Geometry: final body of the model. Coordinates: model frame, mm. Face numbers are marked on the shaded views. A direction names the side the tool comes from. Give positions to 0.01 mm unless a question says otherwise; leave off trailing zeros. Loops run counter-clockwise (first coordinate to the right, second up) from the corner with the lowest first, then second, coordinate; pieces in that order, holes last. Notation, with made-up numbers: (1, 5) -> (32, 5) arc R14 ccw to (32, 23) -> close; hole circle Ø5 at (19.5, 40.5). An arc over 180 degrees is marked (long way). One line per item, written item: value. Start each with the question number.
Autodesk Inventor part; units mm, degrees
ref_plane "YZ Plane" through (0, 0, 0) normal (1, 0, 0) x (0, 1, 0)
ref_plane "XZ Plane" through (0, 0, 0) normal (0, 1, 0) x (-1, 0, 0)
ref_plane "XY Plane" through (0, 0, 0) normal (0, 0, 1) x (1, 0, 0)
sketch "スケッチ1" plane through (0, 0, 0) normal (0, 1, 0) x (-1, 0, 0)
  line L0 (0, 0) -> (-90, 0)
  line L1 (-90, 0) -> (-90, 50)
  line L2 (0, 50) -> (0, 0)
  line L3 (0, 0) -> (-5, 0)
  line L4 (-5, 0) -> (-5, 50)
  line L5 (-5, 0) -> (-90, 0)
  line L6 (-90, 0) -> (-85, 0)
  line L7 (-85, 0) -> (-85, 50)
  arc A0 (-85, 50) -> (-5, 50) centre (-45, 50) ccw
  line L8 (0, 0) -> (0, 10)
  line L9 (0, 10) -> (-90, 10)
  circle A1 centre (-45, 50) radius 45
  line L10 (-90, 5) -> (0, 5)
  line L11 (-90, 50) -> (-85, 50)
  line L12 (-5, 50) -> (0, 50)
  line L13 (0, 0) -> (-90, 0)
  line L14 (-90, 0) -> (-90, 5)
  line L15 (-90, 5) -> (0, 5)
  line L16 (0, 5) -> (0, 0)
  dimension "d0" = 90
  dimension "d1" = 50
  dimension "d2" = 5
  dimension "d3" = 85
  dimension "d4" = 5
  dimension "d5" = 80
  dimension "d6" = 10
  dimension "d7" = 90
extrude "押し出し1" add sketch "スケッチ1" along normal blind 230 contours L0 L4 L10 L2 | L0 L7 L10 L4 | L10 L4 L9 L2 | L0 L1 L10 L7 | L10 A1 L9 L4 | L9 L4 A1 L2 | L10 L1 L9 L7 | L7 L9 A1 L10 | L9 A1 L4 | A1 L9 | A1 L4 L12 | L9 L1 A1 L7 | L7 A1 L9 | A1 L9 A0 L4 | A1 L7 A0 L9 | L11 L7 A1
sketch "スケッチ2" plane through (0, 0, 0) normal (0, -1, 0) x (1, 0, 0)
  line L0 (0, 0) -> (0, 50)
  line L1 (90, 0) -> (0, 0)
  line L2 (90, 50) -> (90, 0)
  line L3 (85, 50) -> (90, 50)
  arc A0 (5, 50) -> (85, 50) centre (45, 50) ccw
  line L4 (0, 50) -> (5, 50)
  arc A1 (5, 23.467) -> (85, 23.467) centre (45, 50) ccw
  line L5 (0, 5) -> (90, 5)
  line L6 (5, 23.467) -> (5, 5)
  line L7 (85, 23.467) -> (85, 5)
  dimension "d29" = 48
extrude "押し出し2" cut sketch "スケッチ2" against normal blind 225 contours L6 A1 L5 | L5 A1 L7
sketch "スケッチ3" plane through (0, 230, 0) normal (0, 1, 0) x (1, 0, 0)
  arc A0 (85, -50) -> (5, -50) centre (45, -50) ccw
  line L0 (90, -50) -> (90, 0)
  line L1 (0, -50) -> (5, -50)
  arc A1 (85, -50) -> (5, -50) centre (45, -50) ccw
  line L2 (5, -50) -> (85, -50)
extrude "押し出し3" add sketch "スケッチ3" against normal blind 5
sketch "スケッチ4" plane through (90, 0, 50) normal (1, 0, 0) x (0, 0, -1)
  line L0 (0, 0) -> (50, 0)
  line L1 (0, 0) -> (0, 230)
  line L2 (25, 0) -> (25, 65)
  line L3 (25, 65) -> (25, 75)
  line L4 (25, 75) -> (25, 215)
  line L5 (25, 215) -> (25, 225)
  line L6 (0, 65) -> (40, 65)
  line L7 (40, 65) -> (40, 75)
  line L8 (40, 75) -> (0, 75)
  line L9 (0, 75) -> (0, 65)
  line L10 (0, 215) -> (40, 215)
  line L11 (40, 215) -> (40, 225)
  line L12 (40, 225) -> (0, 225)
  line L13 (0, 225) -> (0, 215)
  dimension "d16" = 65
  dimension "d17" = 10
  dimension "d18" = 140
  dimension "d19" = 10
  dimension "d20" = 40
extrude "押し出し4" cut sketch "スケッチ4" against normal blind 90 contours L1 L8 L3 L6 | L3 L8 L7 L6 | L1 L12 L5 L10 | L5 L12 L11 L10
sketch "スケッチ6" plane through (90, 0, 50) normal (1, 0, 0) x (0, 0, -1)
  line L0 (0, 230) -> (50, 230)
  line L1 (50, 230) -> (37.5, 251.6506)
  line L2 (50, 230) -> (110, 230) construction
  line L3 (0, 230) -> (37.5, 251.6506)
  line L4 (0, 230) -> (43.3013, 230) construction
  dimension "d32" = 120
  dimension "d33" = 30
extrude "押し出し6" add sketch "スケッチ6" against normal blind 90
sketch "スケッチ9" plane through (0, 0, 0) normal (-1, 0, 0) x (0, 0, 1)
  line L0 (10, 225) -> (50, 225)
  line L1 (50, 225) -> (50, 230)
  line L2 (50, 230) -> (12.5, 251.6506)
  line L3 (12.5, 251.6506) -> (0, 230)
  line L4 (0, 0) -> (0, 230)
  line L5 (0, 0) -> (50, 0)
  line L6 (50, 0) -> (50, 65)
  line L7 (50, 65) -> (10, 65)
  line L8 (10, 65) -> (10, 75)
  line L9 (10, 75) -> (50, 75)
  line L10 (50, 75) -> (50, 215)
  line L11 (50, 215) -> (10, 215)
  line L12 (10, 215) -> (10, 225)
  line L13 (12.5, 251.6506) -> (0, 230)
  line L14 (0, 230) -> (-132.7906, 0)
  line L15 (0, 145) -> (-49.0748, 145)
  line L16 (0, 115) -> (-66.3953, 115)
  dimension "d45" = 30
sketch "スケッチ10" plane through (0, 0, 0) normal (-1, 0, 0) x (0, 0, 1)
  line L0 (10, 225) -> (50, 225)
  line L1 (50, 225) -> (50, 230)
  line L2 (50, 230) -> (12.5, 251.6506)
  line L3 (12.5, 251.6506) -> (0, 230)
  line L4 (0, 0) -> (0, 230)
  line L5 (0, 0) -> (50, 0)
  line L6 (50, 0) -> (50, 65)
  line L7 (50, 65) -> (10, 65)
  line L8 (10, 65) -> (10, 75)
  line L9 (10, 75) -> (50, 75)
  line L10 (50, 75) -> (50, 215)
  line L11 (50, 215) -> (10, 215)
  line L12 (10, 215) -> (10, 225)
  line L13 (12.5, 251.6506) -> (-87.5, 78.4456)
  line L14 (-87.5, 78.4456) -> (50, 0)
sketch "スケッチ12" plane through (90, 0, 50) normal (1, 0, 0) x (0, 0, -1)
  line L0 (50, 0) -> (50, 230)
  line L1 (40, 225) -> (40, 215)
  line L2 (0, 215) -> (0, 75)
  line L3 (0, 145) -> (50, 145)
  line L4 (32.5, 175) -> (17.5, 175)
  line L5 (17.5, 175) -> (17.5, 115)
  line L6 (17.5, 115) -> (32.5, 115)
  line L7 (32.5, 115) -> (32.5, 175)
  line L8 (32.5, 175) -> (17.5, 115) construction
  line L9 (17.5, 175) -> (32.5, 115) construction
  line L10 (17.5, 145) -> (32.5, 145)
  line L11 (32.5, 145) -> (32.5, 115)
  line L12 (32.5, 115) -> (17.5, 115)
  line L13 (17.5, 115) -> (17.5, 145)
  point P0 (25, 145)
  dimension "d59" = 15
  dimension "d60" = 60
extrude "押し出し8" cut sketch "スケッチ12" against normal blind 2.5 contours L3 L7 L6 L5
sketch "スケッチ13" plane through (0, 0, 0) normal (-1, 0, 0) x (0, 0, 1)
  line L0 (0, 0) -> (0, 230)
  line L1 (50, 75) -> (50, 215)
  line L2 (50, 145) -> (0, 145)
  line L3 (17.5, 175) -> (32.5, 175)
  line L4 (32.5, 175) -> (32.5, 115)
  line L5 (32.5, 115) -> (17.5, 115)
  line L6 (17.5, 115) -> (17.5, 175)
  line L7 (17.5, 175) -> (32.5, 115) construction
  line L8 (32.5, 175) -> (17.5, 115) construction
  line L9 (17.5, 145) -> (32.5, 145)
  line L10 (32.5, 145) -> (32.5, 115)
  line L11 (32.5, 115) -> (17.5, 115)
  line L12 (17.5, 115) -> (17.5, 145)
  point P0 (25, 145)
  dimension "d63" = 15
  dimension "d64" = 60
extrude "押し出し9" cut sketch "スケッチ13" against normal blind 2.5 contours L4 L5 L6 L2
sketch "スケッチ14" plane through (90, 0, 0) normal (0, 0, -1) x (-1, 0, 0)
  line L0 (90, 0) -> (90, 230)
  line L1 (0, 0) -> (0, 230)
  line L2 (0, 145) -> (90, 145)
  line L3 (37.5, 170) -> (52.5, 170)
  line L4 (52.5, 170) -> (52.5, 120)
  line L5 (52.5, 120) -> (37.5, 120)
  line L6 (37.5, 120) -> (37.5, 170)
  line L7 (37.5, 170) -> (52.5, 120) construction
  line L8 (52.5, 170) -> (37.5, 120) construction
  line L9 (37.5, 145) -> (52.5, 145)
  line L10 (52.5, 145) -> (52.5, 170)
  line L11 (52.5, 170) -> (37.5, 170)
  line L12 (37.5, 170) -> (37.5, 145)
  point P0 (45, 145)
  dimension "d67" = 15
  dimension "d70" = 25
extrude "押し出し10" cut sketch "スケッチ14" against normal blind 5 contours L6 L3 L4 L2
sketch "スケッチ16" plane through (90, 0, 0) normal (0, 0, -1) x (-1, 0, 0)
  line L0 (52.5, 170) -> (52.5, 145)
  line L1 (52.5, 145) -> (37.5, 145)
  line L2 (37.5, 145) -> (37.5, 170)
  line L3 (90, 0) -> (90, 230)
  line L4 (0, 0) -> (0, 230)
  line L5 (0, 145) -> (90, 145)
  line L6 (0, 160) -> (37.5, 157.5)
  line L7 (52.5, 157.5) -> (90, 157.5)
  line L8 (18.75, 158.75) -> (18.75, 145)
  line L9 (71.25, 145) -> (71.25, 157.5)
  line L10 (11.25, 175) -> (26.25, 175)
  line L11 (26.25, 175) -> (26.25, 115)
  line L12 (26.25, 115) -> (11.25, 115)
  line L13 (11.25, 115) -> (11.25, 175)
  line L14 (11.25, 175) -> (26.25, 115) construction
  line L15 (26.25, 175) -> (11.25, 115) construction
  line L16 (11.25, 115) -> (26.25, 115)
  line L17 (26.25, 115) -> (26.25, 175)
  line L18 (26.25, 175) -> (11.25, 175)
  line L19 (11.25, 175) -> (11.25, 115)
  line L20 (45, 145) -> (45, 125)
  line L21 (78.75, 175) -> (63.75, 175)
  line L22 (63.75, 115) -> (78.75, 115)
  line L23 (78.75, 175) -> (78.75, 115)
  line L24 (63.75, 115) -> (63.75, 175)
  line L25 (63.75, 175) -> (78.75, 175)
  line L26 (78.75, 175) -> (78.75, 115)
  line L27 (78.75, 115) -> (63.75, 115)
  line L28 (63.75, 115) -> (63.75, 175)
  line L29 (11.25, 115) -> (26.25, 115)
  line L30 (26.25, 115) -> (26.25, 175)
  line L31 (26.25, 175) -> (11.25, 175)
  line L32 (11.25, 175) -> (11.25, 115)
  dimension "d71" = 15
  dimension "d72" = 60
  dimension "d73" = 20
extrude "押し出し11" cut sketch "スケッチ16" against normal blind 3 contours L24 L21 L23 L7 | L7 L9 L5 L24 | L5 L23 L22 L24 | L7 L23 L5 L9 | L11 L12 L13 L5 | L5 L8 L6 L11 | L6 L13 L10 L11 | L5 L13 L6 L8
sketch "スケッチ17" plane through (37.5, 145, 0) normal (0, 1, 0) x (1, 0, 0)
  line L0 (-57.7643, 16.522) -> (69.053, 16.522)
  line L1 (69.053, 16.522) -> (69.053, -65.9751)
  line L2 (69.053, -65.9751) -> (-57.7643, -65.9751)
  line L3 (-57.7643, -65.9751) -> (-57.7643, 16.522)
  point P0 (-37.5, 0)
extrude "押し出し12" cut sketch "スケッチ17" against normal blind 180
sketch "スケッチ18" plane through (0, 215, 10) normal (-1, 0, 0) x (0, 0, 1)
  line L0 (-10, -70) -> (40, -70)
  line L1 (7.5, -40) -> (22.5, -40)
  line L2 (22.5, -40) -> (22.5, -100)
  line L3 (22.5, -100) -> (7.5, -100)
  line L4 (7.5, -100) -> (7.5, -40)
  line L5 (7.5, -40) -> (22.5, -100) construction
  line L6 (22.5, -40) -> (7.5, -100) construction
  point P0 (-10, -215)
  point P1 (15, -70)
  dimension "d78" = 15
  dimension "d79" = 60
extrude "押し出し13" add sketch "スケッチ18" against normal blind 2.5
sketch "スケッチ19" plane through (90, 215, 10) normal (1, 0, 0) x (0, 0, -1)
  line L0 (-40, -70) -> (10, -70)
  line L1 (-22.5, -40) -> (-7.5, -40)
  line L2 (-7.5, -40) -> (-7.5, -100)
  line L3 (-7.5, -100) -> (-22.5, -100)
  line L4 (-22.5, -100) -> (-22.5, -40)
  line L5 (-22.5, -40) -> (-7.5, -100) construction
  line L6 (-7.5, -40) -> (-22.5, -100) construction
  point P0 (10, -215)
  point P1 (-15, -70)
  dimension "d82" = 15
  dimension "d83" = 60
extrude "押し出し14" add sketch "スケッチ19" against normal blind 2.5
sketch "スケッチ20" plane through (90, 230, 0) normal (0, 0.5, -0.866) x (-1, 0, 0)
  line L0 (0, 0) -> (0, 25)
  line L1 (0, 0) -> (90, 0)
  line L2 (90, 25) -> (90, 0)
  line L3 (0, 25) -> (90, 25)
  line L4 (0, 12.5) -> (90, 12.5)
  line L5 (45, 12.5) -> (45, 25)
  line L6 (45, 12.5) -> (45, 0)
  line L7 (22.5, 18.5) -> (67.5, 18.5)
  line L8 (67.5, 18.5) -> (67.5, 6.5)
  line L9 (67.5, 6.5) -> (22.5, 6.5)
  line L10 (22.5, 6.5) -> (22.5, 18.5)
  line L11 (22.5, 18.5) -> (67.5, 6.5) construction
  line L12 (67.5, 18.5) -> (22.5, 6.5) construction
  circle A0 centre (45, 6.5) radius 3
  circle A1 centre (67.5, 18.5) radius 3
  circle A2 centre (67.5, 6.5) radius 3
  circle A3 centre (22.5, 6.5) radius 3
  circle A4 centre (22.5, 18.5) radius 3
  circle A5 centre (45, 18.5) radius 3
  point P0 (90, -199.1858)
  dimension "d86" = 45
  dimension "d87" = 6
  dimension "d89" = 6
  dimension "d90" = 6
  dimension "d91" = 6
  dimension "d92" = 6
  dimension "d93" = 6
  dimension "d94" = 6
extrude "押し出し15" add sketch "スケッチ20" along normal blind 5 contours A0 L9 L6 | L6 L9 A0 | A3 L9 L10 | L10 L9 A3 | A4 L7 L10 | L10 L7 A4 | L9 A0 L6 | L6 A0 L9 | A5 L7 L5 | L5 L7 A5 | A5 L7 L5 | L5 L7 A5 | A2 L8 L9 | L9 L8 A2 | A1 L7 L8 | L8 L7 A1
ref_plane "作業平面2" through (45, 160, 50) normal (0, -1, 0) x (1, 0, 0)
sketch "スケッチ21" plane through (45, 160, 50) normal (0, -1, 0) x (1, 0, 0)
  line L0 (-52.9668, 19.8142) -> (54.3752, 19.8142)
  line L1 (54.3752, 19.8142) -> (54.3752, -61.5309)
  line L2 (54.3752, -61.5309) -> (-52.9668, -61.5309)
  line L3 (-52.9668, -61.5309) -> (-52.9668, 19.8142)
  line L4 (-52.9668, 19.8142) -> (54.3752, -61.5309) construction
  line L5 (54.3752, 19.8142) -> (-52.9668, -61.5309) construction
  point P0 (-45, -50)
  point P1 (0.7042, -20.8583)
extrude "押し出し16" cut sketch "スケッチ21" against normal blind 150
sketch "スケッチ22" plane through (90, 115, 32.5) normal (1, 0, 0) x (0, 0, -1)
  line L0 (32.5, 45) -> (-17.5, 45)
  line L1 (15, 30) -> (15, 0)
  line L2 (0, 75) -> (15, 75)
  line L3 (15, 75) -> (15, 15)
  line L4 (15, 15) -> (0, 15)
  line L5 (0, 15) -> (0, 75)
  line L6 (0, 75) -> (15, 15) construction
  line L7 (15, 75) -> (0, 15) construction
  point P0 (32.5, -115)
  point P1 (7.5, 45)
extrude "押し出し17" add sketch "スケッチ22" against normal blind 2.5
sketch "スケッチ23" plane through (0, 115, 17.5) normal (-1, 0, 0) x (0, 0, 1)
  line L0 (32.5, 45) -> (-17.5, 45)
  line L1 (15, 30) -> (15, 0)
  line L2 (0, 75) -> (15, 75)
  line L3 (15, 75) -> (15, 15)
  line L4 (15, 15) -> (0, 15)
  line L5 (0, 15) -> (0, 75)
  line L6 (0, 75) -> (15, 15) construction
  line L7 (15, 75) -> (0, 15) construction
  point P0 (-17.5, -115)
  point P1 (7.5, 45)
extrude "押し出し18" add sketch "スケッチ23" against normal blind 2.5
properties part number "知能ロボコン発射台２.112" material "ABS プラスチック"
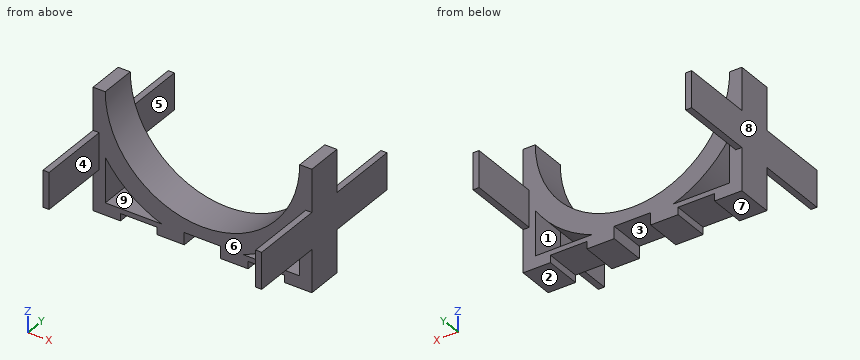
Item 1: Section D-D, the plane z = 14.5. Output: boundary loops of the cut face in (x, y), then the cut area to 3 significant figures.
Item 2: Ray query, line 1 along X through (y, z) = (129, 30); line 2 along Y through (x, z) = (8, 26.5); line 3 along X through (y, z) = (158.5, 13). Return the intervals inside material, ascending. Write a range as [from, to].
Item 3: Section B-B, the plane z = 26. Output: boundary loops of the cut face in (x, y), then the cut area to 3 significant figures.
Item 4: Access query for the marked faces 1, 2, 3, 4 and 5. Directions: +Z, -Z, +X, -X, +Y, -Y. A direction counts if a zero-diameter tool reaches every point of the face in a straight line with its end or side. Return the directions, or none.
Item 5: Pin query (flat end, axial travel): pin 1 (10 mm diameter, centred on x = 66.5, z = 20.5, fed in from -Y); pin 2 (6 mm diameter, centred on x = 43.5, y = 150, fed in from -Z); pin 3 (2 mm diameter, centred on x = 1, y = 171, fed in from -Z); pin 4 (5 mm diameter, centred on x = 75.5, z = 32, fed in from +Y). Return the tip coordinate at first contact, or that it passes through.
Item 6: Section C-C, the plane x = 23.5. Output: boundary loops of the cut face in (y, z).
Item 7: Section A-A, the plane y = 128. Output: boundary loops of the cut face in (x, z), then the cut area to 3 significant figures.
Item 8: Mould query, pull axis X, two halves, no side actions, for the marked faces 6, 7, 8 and 9. Classes: pulls with the +X half, pulls with the -X half, needs draft (parallel to the pull), parting line crosses it, or undercut.
Geometry check:
1. outline: (0, 145) -> (5, 145) -> (5, 160) -> (0, 160) -> close; (12.69, 145) -> (26.57, 145) -> (26.57, 160) -> (12.69, 160) -> close; (63.43, 145) -> (77.31, 145) -> (77.31, 160) -> (63.43, 160) -> close; (85, 145) -> (90, 145) -> (90, 160) -> (85, 160) -> close
1. area: 566 mm2
2. line 1: x = [0, 2.5], [87.5, 90]
2. line 2: y = [145, 160]
2. line 3: x = [0, 5], [14.42, 29.8], [60.2, 75.58], [85, 90]
3. outline: (0, 115) -> (2.5, 115) -> (2.5, 145) -> (13, 145) -> (13, 160) -> (2.5, 160) -> (2.5, 190) -> (0, 190) -> close; (77, 145) -> (87.5, 145) -> (87.5, 115) -> (90, 115) -> (90, 190) -> (87.5, 190) -> (87.5, 160) -> (77, 160) -> close
3. area: 690 mm2
4. face 1: +Y, -Y
4. face 2: -Z, +X, -X, +Y, -Y
4. face 3: -Z, +Y, -Y
4. face 4: +Z, -Z, -Y
4. face 5: +Z, -Z, +Y
5. pin 1: stops at y = 145
5. pin 2: stops at z = 5
5. pin 3: stops at z = 17.5
5. pin 4: passes through
6. outline: (145, 3) -> (160, 3) -> (160, 5) -> (145, 5) -> close; (145, 7.08) -> (160, 7.08) -> (160, 16.27) -> (145, 16.27) -> close
7. outline: (0, 17.5) -> (2.5, 17.5) -> (2.5, 32.5) -> (0, 32.5) -> close; (87.5, 17.5) -> (90, 17.5) -> (90, 32.5) -> (87.5, 32.5) -> close
7. area: 75.0 mm2
8. face 6: undercut
8. face 7: needs draft
8. face 8: pulls with the -X half
8. face 9: undercut
